The model under review builds one solid part; all positions refer to its coordinate system, in mm. Coordinates: 2 decimals unless noted, no trailing zeros. Loops run counter-clockwise (first coordinate to the right, second up) from the corner with the lowest first, then second, coordinate; pieces in that order, holes last. Notation, with made-up numbers: M -15,-28 L 33,-28 A19 ccw 33,-11 Z; hole C -7,-16 d11. An arc over 180 degrees is marked long. One line per item, written item: value.
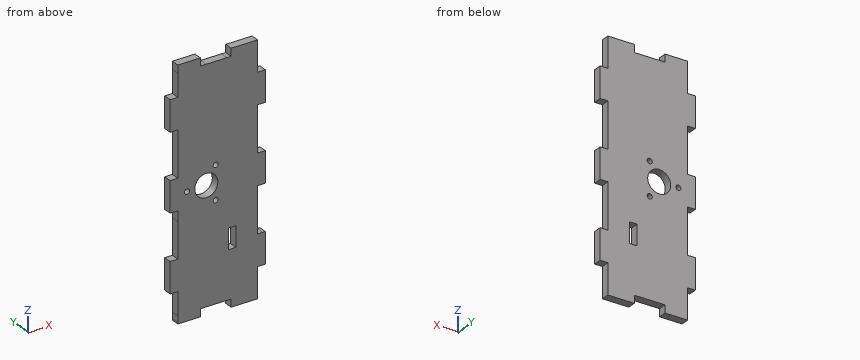
Autodesk Inventor part; units mm, degrees
ref_plane "YZ Plane" through (0, 0, 0) normal (1, 0, 0) x (0, 1, 0)
ref_plane "XZ Plane" through (0, 0, 0) normal (0, 1, 0) x (-1, 0, 0)
ref_plane "XY Plane" through (0, 0, 0) normal (0, 0, 1) x (1, 0, 0)
sketch "Boceto1" plane through (0, 0, 0) normal (0, 1, 0) x (-1, 0, 0)
  line L0 (-13.9366, -26.8506) -> (-11.6866, -26.8506)
  line L1 (-11.6866, -26.8506) -> (-11.6866, -35.7756)
  line L2 (-11.6866, -35.7756) -> (-3.9241, -35.7756)
  line L3 (-3.9241, -35.7756) -> (-3.9241, -33.5256)
  line L4 (-3.9241, -33.5256) -> (5.0759, -33.5256)
  line L5 (5.0759, -33.5256) -> (5.0759, -35.7756)
  line L6 (5.0759, -35.7756) -> (6.7964, -35.7756)
  line L7 (6.7964, -35.7756) -> (11.7134, -35.7756)
  line L8 (11.7134, -35.7756) -> (11.7134, -35.375)
  line L9 (11.7134, -35.375) -> (11.7134, -33.5256)
  line L10 (11.7134, -33.5256) -> (11.7134, -26.8257)
  line L11 (11.7134, -26.8257) -> (13.9634, -26.8257)
  line L12 (13.9634, -26.8257) -> (13.9634, -17.8506)
  line L13 (13.9637, -17.8506) -> (11.7151, -17.8506)
  line L14 (11.7151, -17.8506) -> (11.7144, -7.4795)
  line L15 (11.7144, -7.4795) -> (11.7134, -4.5006)
  line L16 (11.7118, -4.5504) -> (11.7134, -4.5006)
  line L17 (11.7134, -4.5006) -> (13.9634, -4.5006)
  line L18 (13.9634, -4.5006) -> (13.9634, 4.4994)
  line L19 (13.9634, 4.4994) -> (11.7134, 4.4994)
  line L20 (11.7134, 4.4994) -> (11.7134, 17.8494)
  line L21 (11.7134, 17.8494) -> (13.9634, 17.8494)
  line L22 (13.9634, 17.8494) -> (13.9634, 26.8494)
  line L23 (13.9634, 26.8494) -> (11.7134, 26.8494)
  line L24 (11.7134, 26.8494) -> (11.7134, 33.5244)
  line L25 (11.7134, 33.5244) -> (11.7134, 35.7744)
  line L26 (11.7134, 35.7744) -> (5.0759, 35.7744)
  line L27 (5.0759, 35.7744) -> (5.0759, 33.5244)
  line L28 (5.0759, 33.5244) -> (-2.6866, 33.5244)
  line L29 (-2.6866, 33.5244) -> (-3.9241, 33.5244)
  line L30 (-3.9241, 33.5244) -> (-3.9241, 35.7744)
  line L31 (-3.9241, 35.7744) -> (-11.6866, 35.7744)
  line L32 (-11.6866, 35.7744) -> (-11.6866, 26.8494)
  line L33 (-11.6866, 26.8494) -> (-13.9366, 26.8494)
  line L34 (-13.9366, 26.8494) -> (-13.9366, 17.8494)
  line L35 (-13.9366, 17.8494) -> (-11.6866, 17.8494)
  line L36 (-11.6866, 17.8494) -> (-11.6866, 4.4994)
  line L37 (-11.6866, 4.4994) -> (-13.9366, 4.4994)
  line L38 (-13.9366, 4.4994) -> (-13.9366, -4.5006)
  line L39 (-13.9366, -4.5006) -> (-11.6866, -4.5006)
  line L40 (-11.6866, -4.5006) -> (-11.6866, -17.8506)
  line L41 (-11.6866, -17.8506) -> (-13.1866, -17.8506)
  line L42 (-13.1866, -17.8506) -> (-13.9366, -17.8506)
  line L43 (-13.9366, -17.8506) -> (-13.9366, -26.8506)
  line L44 (-12.075, -17.85) -> (-14.325, -17.85)
  line L45 (4.6875, 33.525) -> (3.4125, 33.525)
  line L46 (-3.075, -13.65) -> (-3.075, -19.65)
  line L47 (-3.075, -19.65) -> (-5.325, -19.65)
  line L48 (-5.325, -19.65) -> (-5.325, -13.65)
  line L49 (-5.325, -13.65) -> (-3.075, -13.65)
  circle A0 centre (0.6, 4.875) radius 0.75
  circle A1 centre (3.375, 0) radius 3.375
  circle A2 centre (9, 0) radius 0.75
  circle A3 centre (0.6, -4.875) radius 0.75
  point P0 (0, 0)
extrude "Extrusión1" add sketch "Boceto1" along normal blind 2.4
properties part number "costat3"
(1) Add section B-B on z = 0. State the section outline as (x, y) points.
Checks:
outline: M -13.96,0 L -9.75,0 L -9.75,2.4 L -13.96,2.4 Z; M -8.25,0 L -6.75,0 L -6.75,2.4 L -8.25,2.4 Z; M 0,0 L 13.94,0 L 13.94,2.4 L 0,2.4 Z
(2) Add section C-C on y = 1.6. State how many separate pieces and enclosed holes the cut face has, then the cut area to 3 significant figures.
Checks:
separate pieces: 1
enclosed holes: 5
area: 1,700 mm^2
(3) Insertion check: pin 1 Ø1.1 at (x, y) = (12.5, 1) entering from -Z; pin 2 Ø1.5 at (x, z) = (10.5, 11) entering from -Y; pin 3 Ø0.7 at (x, y) = (-13, 1) entering from -Z. Each pin has a flat end and moves straight along its axis. Give the tip position at first contact, or say it passes through.
Checks:
pin 1: z = -26.85
pin 2: y = 0
pin 3: z = -26.83
(4) To check wall thickness, follow L1, parallel to X at y = 2, z = -16.5 (3 decimals); L2, parallel to Z at x = -9, y = 0.4; L3, parallel to Z at x = -0.75, y = 0.5. State the ranges of each line that lie inside material, in increasing order. Write a range as [from, to].
Checks:
L1: [-11.715, 3.075], [5.325, 11.687]
L2: [-35.78, -0.75], [0.75, 35.77]
L3: [-33.53, -5.61], [-4.14, -2.12], [2.12, 4.14], [5.61, 33.52]
(5) Add section A-A on x = -9. State the section outline as (y, z) points, then the cut area to 3 significant figures.
Checks:
outline: M 0,-35.78 L 2.4,-35.78 L 2.4,-0.75 L 0,-0.75 Z; M 0,0.75 L 2.4,0.75 L 2.4,35.77 L 0,35.77 Z
area: 168 mm^2
